from build123d import *

# Parameters (mm, degrees)
BOSS_EXTRUDE1_DEPTH = 2
BOSS_EXTRUDE2_DEPTH = 3
FILLET1_R           = 5
FILLET2_R           = 0.5


with BuildPart() as part:
    # Sketch1 → Boss-Extrude1 (new body)
    with BuildSketch(Plane(origin=(0, 0, 0), x_dir=(1, 0, 0), z_dir=(0, 1, 0))):
        Polygon((0, 0), (0, 45), (45, 0), align=None)
    extrude(amount=BOSS_EXTRUDE1_DEPTH)

    # Sketch2 → Boss-Extrude2 (add)
    with BuildSketch(Plane(origin=(0, 2, 0), x_dir=(1, 0, 0), z_dir=(0, 1, 0))):
        Polygon((2, 43), (2, 2), (43, 2), (45, 0), (0, 0), (0, 45), align=None)
    extrude(amount=BOSS_EXTRUDE2_DEPTH)

    # Fillet1
    fillet1_edges = [part.edges().sort_by_distance(p)[0] for p in [
        (0, 0, -22.5),
        (22.5, 0, 0),
        (45, 2.5, 0),
        (0, 2.5, -45),
    ]]
    fillet(fillet1_edges, radius=FILLET1_R - 0.0001)  # a hair under: the kernel refuses the full size

    # Fillet2
    fillet2_edges = [part.edges().sort_by_distance(p)[0] for p in [
        (36.929123609, 3.5, -2),
        (2, 3.5, -36.929123609),
    ]]
    fillet(fillet2_edges, radius=FILLET2_R)


solid = part.part
Source: CAD feature listing. Evaluate the final solid. Frame: model axes, mm. A direction names the side the tool comes from. Round coordinates to 2 decimals unless told otherwise and drop trailing zeros. Loops run counter-clockwise (first coordinate to the right, second up) from the corner with the lowest first, then second, coordinate; pieces in that order, holes last. Notation, with made-up numbers: (7, 35.25) - (49, 35.25) arc R26 cw to (49, 74.25) - close; hole circle Ø9 at (0.5, 0). An arc over 180 degrees is marked (long way). Write item = value, one per line. Start each with the question number.
(1) Pin query (flat end, axial travel): pin 1 (1 mm diameter, centred on y = 3, z = -12, fed in from +X); pin 2 (1 mm diameter, centred on y = 4, z = -6, fed in from -X); pin 3 (2 mm diameter, centred on x = 33, y = 3.5, fed in from -Z). Return the tip coordinate at first contact, or that it passes through.
(2) Set-up query: faces 1 (the face through (1.675, 3.479, -36.226)), 2 (the face through (19, 3, -2)), 3 (the face through (36.226, 3.479, -1.675)). Return all of +Z, -Z, +X, -X, +Y, -Y with unobstructed straight access to the full face (end or side cutting, diameter ignored); none if empty.
(3) Ray query, line 1 along Y through (x, z) = (23, -20.5); line 2 along X through (y, z) = (2.4, -14); line 3 along Z through (x, y) = (18.5, 1.05). Return the intervals inside material, ascending. Write a range as from..to.
(4) Section query C-C, the plane y = 2.75. Output: boundary loops of the cut face in (x, z).
Conclusion:
q1.pin_1 = 2
q1.pin_2 = 0.03
q1.pin_3 = -2
q2.face_1 = -Z, +Y
q2.face_2 = -Z, +X, +Y
q2.face_3 = +X, +Y
q3.line_1 = 0..2
q3.line_2 = 0.73..2
q3.line_3 = -26.5..-1.93
q4.outline = (0.53, -35.18) arc R5 ccw to (1.11, -36.07) arc R0.5 ccw to (2, -35.76) - (2, -2) - (35.76, -2) arc R0.5 ccw to (36.07, -1.11) arc R5 ccw to (35.18, -0.53) - (0.53, -0.53) - close
